Geometry: final body of the model. Coordinates: model frame, mm. A direction names the side the tool comes from. Give positions to 0.01 mm unless a question says otherwise; leave off trailing zeros. Order: outer loops, then holes, each group sorted by start corner. A loop starts at its lowest first (then second) coordinate and runs counter-clockwise, first axis right, second up. Notation, with made-up numbers: (64.25, 12) -> (108.25, 12) arc R7 cw to (108.25, 22) -> close; hole circle Ø10 at (63, 51). An arc over 180 degrees is marked (long way). One line per item, written item: value. Start each with the question number.
```python
from build123d import *

# Parameters (mm, degrees)
CORTAR_EXTRUIR1_DEPTH      = 231.52548666
CORTAR_EXTRUIR1_DEPTH_BACK = 231.52548666
CROQUIS2_R                 = 4.7625
CHAFL_N1_SIZE              = 1.5


with BuildPart() as part:
    # Croquis1 → Revolución1 (revolve)
    with BuildSketch(Plane.XY, mode=Mode.PRIVATE) as revoluci_n1_sk:
        Polygon((0, 0), (7.5, 12.990381057), (7.5, 30), (9.525, 30), (9.525, 187), (7.5, 187), (7.5, 192), (11, 192), (11, 230), (0, 230), align=None)
    revolve(revoluci_n1_sk.sketch.rotate(Axis((0, 0, 0), (0, 1, 0)), 90), axis=Axis((0, 0, 0), (0, 1, 0)))

    # Croquis2 → Cortar-Extruir1 (cut, two sides: drawn at the far end of the back side and taken through both)
    with BuildSketch(Plane.XY.offset(-CORTAR_EXTRUIR1_DEPTH_BACK)):
        with Locations((0, 211)):
            Circle(CROQUIS2_R)
    extrude(amount=CORTAR_EXTRUIR1_DEPTH + CORTAR_EXTRUIR1_DEPTH_BACK, mode=Mode.SUBTRACT)

    # Chaflán1
    chafl_n1_edges = [part.edges().sort_by_distance(p)[0] for p in [
        (0, 230, 11),
    ]]
    chamfer(chafl_n1_edges, length=CHAFL_N1_SIZE)


solid = part.part
```
1. Access query for faces 1 (the cylindrical face through (-6.324, 21.614, -4.032)), 2 (the flat face through (0, 230, 0)), 3 (the flat face through (8, 187, 0)). Directions: +Z, -Z, +X, -X, +Y, -Y. A direction counts if a zero-diameter tool reaches every point of the face in a straight line with its end or side. Return the directions, or none.
2. Draft query along Y for faces 4 (the flat face through (8, 30, 0)), 5 (the cylindrical face through (4.4, 209.18, -0.15)), 6 (the cylindrical face through (9.3, 109.6, 2.06)), 7 (the cylindrical face through (-6.324, 189.535, -4.032)). Return one class per face: pulls with the +Y half, pulls with the -Y half, needs draft (parallel to the pull), parting line crosses it, or undercut.
3. Pin query (flat end, axial travel): P1, Ø2, axis at y = 54.5, z = 7, coming from the -X side; P2, Ø10, axis at y = 76, z = -5, coming from the +X side (3 decimals); P3, Ø6, axis at x = -2.5, z = 2, coming from the -Y side; P4, Ø5.5, axis at x = 0, y = 211, coming from the +Z side. Return the tip coordinate at first contact, or that it passes through.
4. Cut plane B-B, the plane y = 66.5. Return loops of the section in (x, z) (3 decimals), then the cut area to 3 significant figures.
5. Material intervals for L1, parallel to Z at x = -0.25, y = 95.5; L2, parallel to Z at x = -0.75, y = 29.5; L3, parallel to Y at x = 1.5, z = 3.75, sorted ascending. Write a range as [from, to].
6. Cut plane A-A, the plane y = 211. Return loops of the section in (x, z).
Answers follow:
1. face 1: -Y
1. face 2: +Z, -Z, +X, -X, +Y
1. face 3: none
2. face 4: pulls with the -Y half
2. face 5: undercut
2. face 6: needs draft
2. face 7: undercut
3. P1: stops at x = -7.4
3. P2: stops at x = 9.525
3. P3: stops at y = 0.35
3. P4: passes through
4. outline: circle Ø19.05 at (0, 0)
4. area: 285 mm²
5. L1: z = [-9.52, 9.52]
5. L2: z = [-7.46, 7.46]
5. L3: y = [7, 206.48], [215.52, 230]
6. outline: (-4.76, -9.92) -> (-4.76, 9.92) arc R11 ccw to start; (4.76, -9.92) arc R11 ccw to (4.76, 9.92) -> close
